The figure shows three views and two pictorial views of one solid part (mm, origin at its lowest corner). Answer the questions. Coordinates: 2 decimals unless noted, no trailing zeros. Order: outer loops, then holes, each group sorted by start corner. A loop starts at its lowest first (then second) coordinate and runs counter-clockwise, first axis right, second up. Notation, with made-up numbers: M -10,85.25 L 36,85.25 A16 ccw 36,110.25 Z; hole C 51.25,40 d8. An arc over 180 degrees is marked long. Write item = value, one per line. Start each with the question number.
Q1. Find section B-B on x = 24. Give the vertices of the cut face in (y, z).
Q2. Straight lines are drawn through the part: line 1 along X through (y, z) = (5.5, 53.5); line 2 along X through (y, z) = (2.5, 68.58); line 3 along Z through (x, y) = (57, 2). For each, find the intervals that lie inside material, in ascending order.
Q3. Find section C-C on z = 46.5. Give the vertices of the cut face in (x, y).
Q4. Find section D-D on y = 5. Give the vertices of the cut face in (x, z) (3 decimals), and give its area (3 significant figures).
Q5. Find section A-A on z = 7.62. Give the vertices of the cut face in (x, y).
Q6. This flat-tipped pin is pushed along its axis until it touches: P1, Ø5.5, axis at x = 22.098, z = 7.62, coming from the +Y side. Where does it stop, or does it pass through?
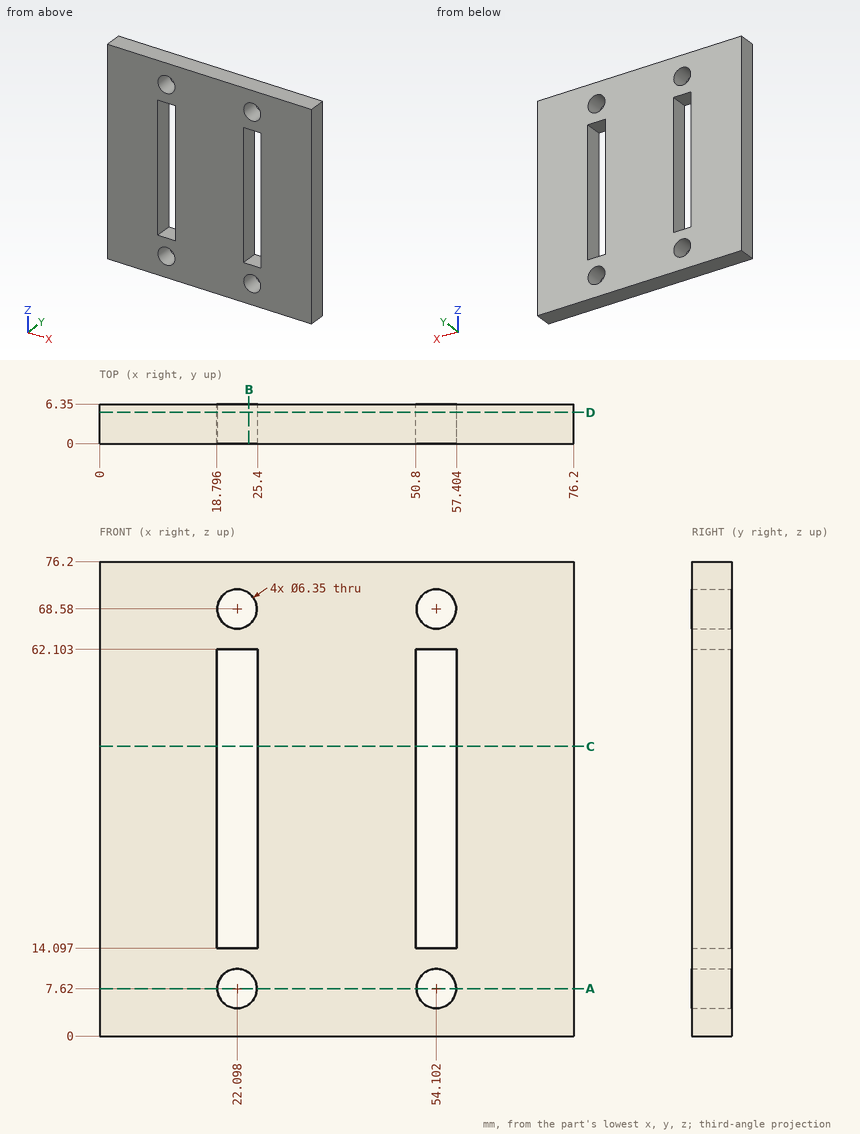
Findings below:
q1.outline = M 0,0 L 6.35,0 L 6.35,5.08 L 0,5.08 Z; M 0,10.16 L 6.35,10.16 L 6.35,14.1 L 0,14.1 Z; M 0,62.1 L 6.35,62.1 L 6.35,66.04 L 0,66.04 Z; M 0,71.12 L 6.35,71.12 L 6.35,76.2 L 0,76.2 Z
q2.line_1 = 0 to 18.8, 25.4 to 50.8, 57.4 to 76.2
q2.line_2 = 0 to 18.92, 25.27 to 50.93, 57.28 to 76.2
q2.line_3 = 0 to 6.32, 8.92 to 14.1, 62.1 to 67.28, 69.88 to 76.2
q3.outline = M 0,0 L 18.8,0 L 18.8,6.35 L 0,6.35 Z; M 25.4,0 L 50.8,0 L 50.8,6.35 L 25.4,6.35 Z; M 57.4,0 L 76.2,0 L 76.2,6.35 L 57.4,6.35 Z
q4.outline = M 0,0 L 76.2,0 L 76.2,76.2 L 0,76.2 Z; hole M 18.796,14.097 L 25.4,14.097 L 25.4,62.103 L 18.796,62.103 Z; hole C 22.098,7.62 d6.35; hole C 22.098,68.58 d6.35; hole M 50.8,14.097 L 57.404,14.097 L 57.404,62.103 L 50.8,62.103 Z; hole C 54.102,7.62 d6.35; hole C 54.102,68.58 d6.35
q4.area = 5,050 mm^2
q5.outline = M 0,0 L 18.92,0 L 18.92,6.35 L 0,6.35 Z; M 25.27,0 L 50.93,0 L 50.93,6.35 L 25.27,6.35 Z; M 57.28,0 L 76.2,0 L 76.2,6.35 L 57.28,6.35 Z
q6.P1 = through
